Part model, mm, in its own coordinate system. A direction names the side the tool comes from. Give positions to 0.01 mm unless a question says otherwise; leave off trailing zeros. Order: outer loops, then holes, each group sorted by start corner. A loop starts at its lowest first (then second) coordinate and runs counter-clockwise, first axis right, second up. Notation, with made-up numbers: (63, -2.75) - (96, -2.75) arc R33 cw to (96, 26.25) - close; hole circle Ø4 at (1, -34.5). An arc over 180 degrees is marked (long way). One line per item, written item: value.
```python
from build123d import *

# Parameters (mm, degrees)
SKETCH1_W           = 115
SKETCH1_H           = 31
BOSS_EXTRUDE1_DEPTH = 19
SHELL1_T            = 5
SKETCH2_R           = 1.5
CUT_EXTRUDE1_DEPTH  = 19
SKETCH3_W           = 10
SKETCH3_H           = 5
BOSS_EXTRUDE2_DEPTH = 10
SKETCH4_R           = 1.5
CUT_EXTRUDE2_DEPTH  = 127.716218378


with BuildPart() as part:
    # Sketch1 → Boss-Extrude1 (new body)
    with BuildSketch(Plane.XY):
        with Locations((57.5, 15.5)):
            Rectangle(SKETCH1_W, SKETCH1_H)
    extrude(amount=BOSS_EXTRUDE1_DEPTH)

    # Shell1
    shell1_openings = [part.faces().sort_by_distance(p)[0] for p in [
        (57.5, 15.5, 19),
    ]]
    offset(amount=SHELL1_T, openings=shell1_openings, kind=Kind.INTERSECTION)

    # Sketch2 → Cut-Extrude1 (cut)
    with BuildSketch(Plane(origin=(120, 0, 0), x_dir=(0, 0, -1), z_dir=(1, 0, 0))):
        with Locations((-7, 15.5)):
            Circle(SKETCH2_R)
    extrude(amount=-CUT_EXTRUDE1_DEPTH, mode=Mode.SUBTRACT)

    # Sketch3 → Boss-Extrude2 (add)
    with BuildSketch(Plane(origin=(0, -5, 0), x_dir=(-1, 0, 0), z_dir=(0, -1, 0))):
        with Locations((0, -16.5)):
            Rectangle(SKETCH3_W, SKETCH3_H)
        with Locations((-115, -16.5)):
            Rectangle(SKETCH3_W, SKETCH3_H)
    extrude(amount=BOSS_EXTRUDE2_DEPTH)

    # Sketch4 → Cut-Extrude2 (cut, through all)
    with BuildSketch(Plane(origin=(0, 0, 14), x_dir=(-1, 0, 0), z_dir=(0, 0, -1))):
        with Locations((0, -10)):
            Circle(SKETCH4_R)
        with Locations((-115, -10)):
            Circle(SKETCH4_R)
    extrude(amount=-CUT_EXTRUDE2_DEPTH, mode=Mode.SUBTRACT)


solid = part.part
```
1) Slice it at B-B on z = 1.75. Write the cut outline in (x, y), then the cut area to 3 significant figures.
Answer:
outline: (-5, -5) - (120, -5) - (120, 36) - (-5, 36) - close; hole (0, 0) - (115, 0) - (115, 31) - (0, 31) - close
area: 1,560 mm2
2) Drop flat-ended pins along their axis: P1, Ø12, axis at x = 47, z = 1.5, coming from the -Y side; P2, Ø15.5, axis at x = 68.5, y = 13.5, coming from the +Z side; P3, Ø3, axis at x = 1.5, y = -8, coming from the -Z side. Give the stop position or say it passes through.
Answer:
P1: stops at y = -5
P2: stops at z = 0
P3: stops at z = 14
3) Two-plate mould, pull along Y, no slides. Class faces 6 (the face through (110, -10, 17)), 7 (the face through (116.5, -9.93, 16.46)), 8 (the face through (0, -15, 16)): pulls with the +Y half, pulls with the -Y half, needs draft (parallel to the pull), parting line crosses it, or undercut.
Answer:
face 6: needs draft
face 7: undercut
face 8: pulls with the -Y half
4) Wall check: line 1 along Y through (x, z) = (59, 17); line 2 along X through (y, z) = (27, 7.25); line 3 along Y through (x, z) = (116.75, 7). Give the ranges that are in metal, low to high. Write a range as [from, to].
Answer:
line 1: y = [-5, 0], [31, 36]
line 2: x = [-5, 0], [115, 120]
line 3: y = [-5, 14], [17, 36]
5) Slice it at D-D on z = 7. Write the cut outline in (x, y).
Answer:
outline: (-5, -5) - (120, -5) - (120, 14) - (115, 14) - (115, 0) - (0, 0) - (0, 31) - (115, 31) - (115, 17) - (120, 17) - (120, 36) - (-5, 36) - close
6) Slice it at C-C on x = 35. Write the cut outline in (y, z), then the cut area to 3 significant figures.
Answer:
outline: (-5, -5) - (36, -5) - (36, 19) - (31, 19) - (31, 0) - (0, 0) - (0, 19) - (-5, 19) - close
area: 395 mm2
7) Slice it at A-A on y = -10. Write the cut outline in (x, z).
Answer:
outline: (-5, 14) - (-1.5, 14) - (-1.5, 19) - (-5, 19) - close; (1.5, 14) - (5, 14) - (5, 19) - (1.5, 19) - close; (110, 14) - (113.5, 14) - (113.5, 19) - (110, 19) - close; (116.5, 14) - (120, 14) - (120, 19) - (116.5, 19) - close
8) Which spindle directions (+Z, -Z, +X, -X, +Y, -Y) get a long thin tool onto all of the face, cutting with end or side? Do faces 1 (the face through (5, -10, 17)), 2 (the face through (1.2, -8.8, 14)), 3 (the face through (57, 0, 9)), 4 (the face through (0.325, -11.464, 16.465)), 5 (the face through (117.54, 15.57, 8.5)). Say none if no direction does.
Answer:
face 1: +Z, -Z, -Y
face 2: -Z, +X, -X, -Y
face 3: +Z
face 4: +Z, -Z
face 5: +X
